from build123d import *

# Parameters (mm, degrees)
FILLET1_R       = 0.2
CHAMFER1_SIZE   = 0.181209408
CHAMFER1_SIZE_2 = 0.05


with BuildPart() as part:
    # Sketch1 → Revolve1 (revolve)
    with BuildSketch(Plane.XY):
        with BuildLine():
            Line((-6, -5), (-6, 5))
            Line((-6, 5), (-7.483314774, 5))
            ThreePointArc((-7.483314774, 5), (-9, 0), (-7.483314774, -5))
            Line((-7.483314774, -5), (-6, -5))
        make_face()
    revolve(axis=Axis((0, 0, 0), (0, 1, 0)))

    # Fillet1
    fillet1_edges = [part.edges().sort_by_distance(p)[0] for p in [
        (6, 5, 0),
        (6, -5, 0),
    ]]
    fillet(fillet1_edges, radius=FILLET1_R)

    # Chamfer1
    # the kernel refuses this chamfer: 0.181209408, 0.05 mm, written as the material it takes off along each edge
    with BuildSketch(Plane(origin=(0, -5, 0), x_dir=(-1, 0, 0), z_dir=(0, 0, -1))) as chamfer1_piece_1:
        with BuildLine():
            Line((7.483314774 - CHAMFER1_SIZE, 0), (7.510900969, 0.041535859))
            ThreePointArc((7.510900969, 0.041535859), (7.49854981, 0.022877263), (7.483314774, 0))
            Line((7.483314774, 0), (7.483314774 - CHAMFER1_SIZE, 0))
        make_face()
    revolve(axis=Axis((0, -5, 0), (0, 1, 0)), mode=Mode.SUBTRACT)
    with BuildSketch(Plane(origin=(0, 5, 0), x_dir=(-1, 0, 0), z_dir=(0, 0, -1))) as chamfer1_piece_2:
        with BuildLine():
            Line((7.577969598, -0.144654824), (7.483314774 - CHAMFER1_SIZE_2, 0))
            Line((7.483314774 - CHAMFER1_SIZE_2, 0), (7.483314774, 0))
            ThreePointArc((7.483314774, 0), (7.532931313, -0.075068951), (7.577969598, -0.144654824))
        make_face()
    revolve(axis=Axis((0, 5, 0), (0, 1, 0)), mode=Mode.SUBTRACT)


solid = part.part
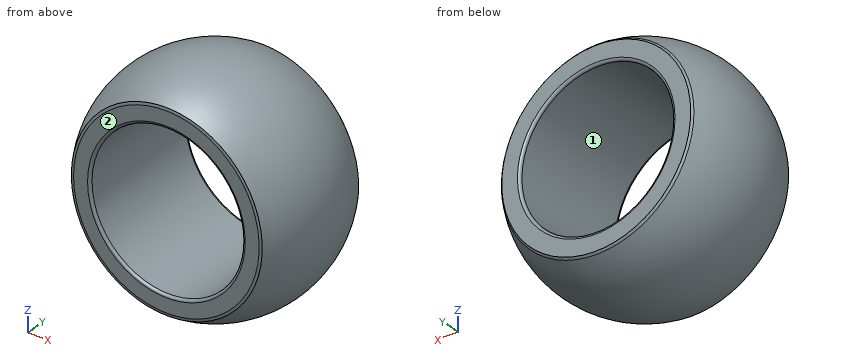
Check sheet for the modelled part. Datum: model origin and axes. Units: mm. Face numbers are marked on the shaded views. Round coordinates to 2 decimals unless told otherwise and drop trailing zeros. Order: outer loops, then holes, each group sorted by start corner. A loop starts at its lowest first (then second) coordinate and runs counter-clockwise, first axis right, second up.
(1) Cross-section at C-C, the plane y = -4. Enter the section's corners in (x, z).
(2) Cross-section at B-B, the plane z = 0. Enter the section's corners in (x, y).
(3) Go/stop test with flat-tipped pins: P1, Ø1.5, axis at y = -2, z = -0.5, coming from the -X side; P2, Ø4, axis at y = -3, z = -5.5, coming from the +X side; P3, Ø6, axis at y = 3.5, z = 6.5, coming from the -X side. Record where each tip stops, or that it passes through.
(4) Draft check along X on the marked faces 1 and 2. Enter one of: pulls with the +X half, pulls with the -X half, needs draft (parallel to the pull), parting line crosses it, or undercut.
(5) Scan lines: probe 1 along Z at (x, y) = (0, -2.25); probe 2 along Z at (x, y) = (0, 0.25); probe 3 along X at (y, z) = (-1.25, 5.25). Record each from-to range of solid material in increasing order.
(6) Cross-section at D-D, the plane y = -0.5. Enter the section's corners in (x, z).
(7) Cross-section at A-A, the plane x = 0. Enter the section's corners in (y, z), and give its area (3 significant figures).
Check sheet entries:
1. outline: circle Ø16.12 at (0, 0); hole circle Ø12 at (0, 0)
2. outline: (-7.58, 4.86) arc R9 ccw to (-7.51, -4.96) - (-7.3, -5) - (-6.2, -5) arc R0.2 ccw to (-6, -4.8) - (-6, 4.8) arc R0.2 ccw to (-6.2, 5) - (-7.43, 5) - close; (6, -4.8) arc R0.2 ccw to (6.2, -5) - (7.3, -5) - (7.51, -4.96) arc R9 ccw to (7.58, 4.86) - (7.43, 5) - (6.2, 5) arc R0.2 ccw to (6, 4.8) - close
3. P1: stops at x = -8.9
3. P2: stops at x = 7.93
3. P3: stops at x = -7.86
4. face 1: undercut
4. face 2: needs draft
5. probe 1: z = -8.71 to -6, 6 to 8.71
5. probe 2: z = -9 to -6, 6 to 9
5. probe 3: x = -7.2 to -2.9, 2.9 to 7.2
6. outline: circle Ø17.97 at (0, 0); hole circle Ø12 at (0, 0)
7. outline: (-5, -7.3) - (-4.96, -7.51) arc R9 ccw to (4.86, -7.58) - (5, -7.43) - (5, -6.2) arc R0.2 ccw to (4.8, -6) - (-4.8, -6) arc R0.2 ccw to (-5, -6.2) - close; (-5, 6.2) arc R0.2 ccw to (-4.8, 6) - (4.8, 6) arc R0.2 ccw to (5, 6.2) - (5, 7.43) - (4.86, 7.58) arc R9 ccw to (-4.96, 7.51) - (-5, 7.3) - close
7. area: 50.2 mm2
